The model under review builds one solid part; all positions refer to its coordinate system, in mm. A direction names the side the tool comes from. Coordinates: 2 decimals unless noted, no trailing zeros. Write each loop counter-clockwise with the first axis right and the second up, starting at its lowest first coordinate (ties: lowest second). Pieces come first, ordered by that corner, then holes.
1) Mouldability with a two-part tool opening along Y and no side actions: class faces 1 (the flat face through (-39, 7.537, 1)), 2 (the cylindrical face through (-42.1, 27.1, 0.5)), 3 (the flat face through (-40.387, 20, 8)) as released by +Y, released by -Y, zero draft, split by the parting line, or undercut.
2) Machinability: for faces 4 (the cylindrical face through (-42.11, 28, -1.78)), 5 (the flat face through (-40, 14, 0)), 6 (the cylindrical face through (-42.113, 25.412, 10.452)), 7 (the flat face through (-42, 13.633, 8)), 8 (the flat face through (-37, 15.537, 1)), which of the approach directions +Z, -Z, +X, -X, +Y, -Y give a long, thin tool a straight path to every point of the face, cutting with its end or side? Answer none if there is none.
3) Add section D-D, the plane x = -39.75. State the section outline as (y, z) points.
4) Add section C-C, the plane z = -0.5. State the section outline as (x, y) points, then the cut area to 3 significant figures.
5) For line 1 (Z direction, x = -36.5, y = 13.75); line 2 (Y direction, x = -42.5, z = 3); line 3 (Y direction, x = -37.75, z = 0.5), list the stretches that pass through material, from the lowest coordinate up.
6) For P1, Ø3, axis at x = -42, z = 5.5, coming from the -Y side; P2, Ø5, axis at y = 26.5, z = 11, coming from the +X side; P3, Ø1, axis at x = -36.5, z = 1.5, coming from the +Y side; P4, Ø2.5, axis at x = -37.39, y = 12.04, coming from the +Z side, all flat-tipped, find the tip position at first contact; note any pin that passes through.
7) Add section A-A, the plane y = 27. State the section outline as (x, z) points.
8) Add section B-B, the plane x = -36.75. State the section outline as (y, z) points, then the cut area to 3 significant figures.
from build123d import *

# Parameters (mm, degrees)
CROQUIS1_W                   = 26
CROQUIS1_H                   = 28
CROQUIS1_R                   = 1.5
SALIENTE_EXTRUIR1_DEPTH      = 2
CROQUIS7_W                   = 3
CROQUIS7_H                   = 8
SALIENTE_EXTRUIR3_DEPTH      = 2
SALIENTE_EXTRUIR2_DEPTH      = 3
SALIENTE_EXTRUIR2_DEPTH_BACK = 0.5
CORTAR_EXTRUIR1_DEPTH        = 2


with BuildPart() as part:
    # Croquis1 → Saliente-Extruir1 (new body)
    with BuildSketch(Plane.XY):
        with Locations((-27.887270297, 1.536585366)):
            Rectangle(CROQUIS1_W, CROQUIS1_H)
        with Locations((-37.387270297, 12.036585366)):
            Circle(CROQUIS1_R, mode=Mode.SUBTRACT)
        with Locations(Location((-18.387270297, 12.036585366, 0), (0, 0, 180))):
            Circle(CROQUIS1_R, mode=Mode.SUBTRACT)
        with Locations((-27.887270297, -5.463414634)):
            Circle(CROQUIS1_R, mode=Mode.SUBTRACT)
    extrude(amount=SALIENTE_EXTRUIR1_DEPTH)

    # Croquis7 → Saliente-Extruir3 (add)
    with BuildSketch(Plane.XY.offset(2)):
        with Locations((-42.387270297, 11.536585366)):
            Rectangle(CROQUIS7_W, CROQUIS7_H)
    extrude(amount=-SALIENTE_EXTRUIR3_DEPTH)

    # Croquis4 → Saliente-Extruir2 (add, two sides: drawn at the far end of the back side and taken through both)
    with BuildSketch(Plane.ZY.offset(40.887270297).offset(-SALIENTE_EXTRUIR2_DEPTH_BACK)):
        with BuildLine():
            Line((0, 15.536585366), (0, 23.686563701))
            ThreePointArc((0, 23.686563701), (-1.75950275, 28.072068742), (2, 30.934697509))
            ThreePointArc((2, 30.934697509), (11.897715698, 27.332223608), (17.164180221, 18.210439479))
            ThreePointArc((17.164180221, 18.210439479), (16.311003312, 15.026339908), (13.323429984, 13.633211586))
            Line((13.323429984, 13.633211586), (2, 13.633211586))
            Line((2, 13.633211586), (2, 15.536585366))
            Line((2, 15.536585366), (0, 15.536585366))
        make_face()
        with BuildLine():
            ThreePointArc((14.800641614, 17.793683853), (10.355025435, 25.493716944), (2, 28.534697509))
            ThreePointArc((2, 28.534697509), (0.5, 27.034697509), (2, 25.534697509))
            ThreePointArc((2, 25.534697509), (8.426662606, 23.195583615), (11.846218354, 17.27273932))
            ThreePointArc((11.846218354, 17.27273932), (13.583902251, 16.055999957), (14.800641614, 17.793683853))
        make_face(mode=Mode.SUBTRACT)
    extrude(amount=SALIENTE_EXTRUIR2_DEPTH + SALIENTE_EXTRUIR2_DEPTH_BACK)

    # Croquis5 → Cortar-Extruir1 (cut)
    with BuildSketch(Plane.XY.offset(2)):
        Polygon((-34.387270297, 15.536585366), (-34.387270297, 7.536585366), (-40.887270297, 7.536585366), (-40.887270297, -12.463414634), (-14.887270297, -12.463414634), (-14.887270297, 15.536585366), align=None)
    extrude(amount=-CORTAR_EXTRUIR1_DEPTH, mode=Mode.SUBTRACT)


solid = part.part
Geometry results:
1. face 1: released by -Y
1. face 2: undercut
1. face 3: zero draft
2. face 4: -Z, +X, -X
2. face 5: -Z, +X, -X, -Y
2. face 6: +X, -X
2. face 7: +Z, +X, -X, -Y
2. face 8: +Z, -Z, +X, +Y
3. outline: (7.54, 0) - (15.54, 0) - (15.54, 2) - (7.54, 2) - close
4. outline: (-43.89, 24.04) - (-40.39, 24.04) - (-40.39, 30.03) - (-43.89, 30.03) - close
4. area: 21.0 mm2
5. line 1: z = 0 to 2
5. line 2: y = 13.63 to 25.48, 28.5 to 30.9
5. line 3: y = 7.54 to 10.58, 13.49 to 15.54
6. P1: stops at y = 13.63
6. P2: stops at x = -40.39
6. P3: stops at y = 15.54
6. P4: passes through
7. outline: (-43.89, -1.9) - (-40.39, -1.9) - (-40.39, 0.5) - (-43.89, 0.5) - close; (-43.89, 8.13) - (-40.39, 8.13) - (-40.39, 12.28) - (-43.89, 12.28) - close
8. outline: (7.54, 0) - (10.68, 0) - (10.68, 2) - (7.54, 2) - close; (13.39, 0) - (15.54, 0) - (15.54, 2) - (13.39, 2) - close
8. area: 10.6 mm2
